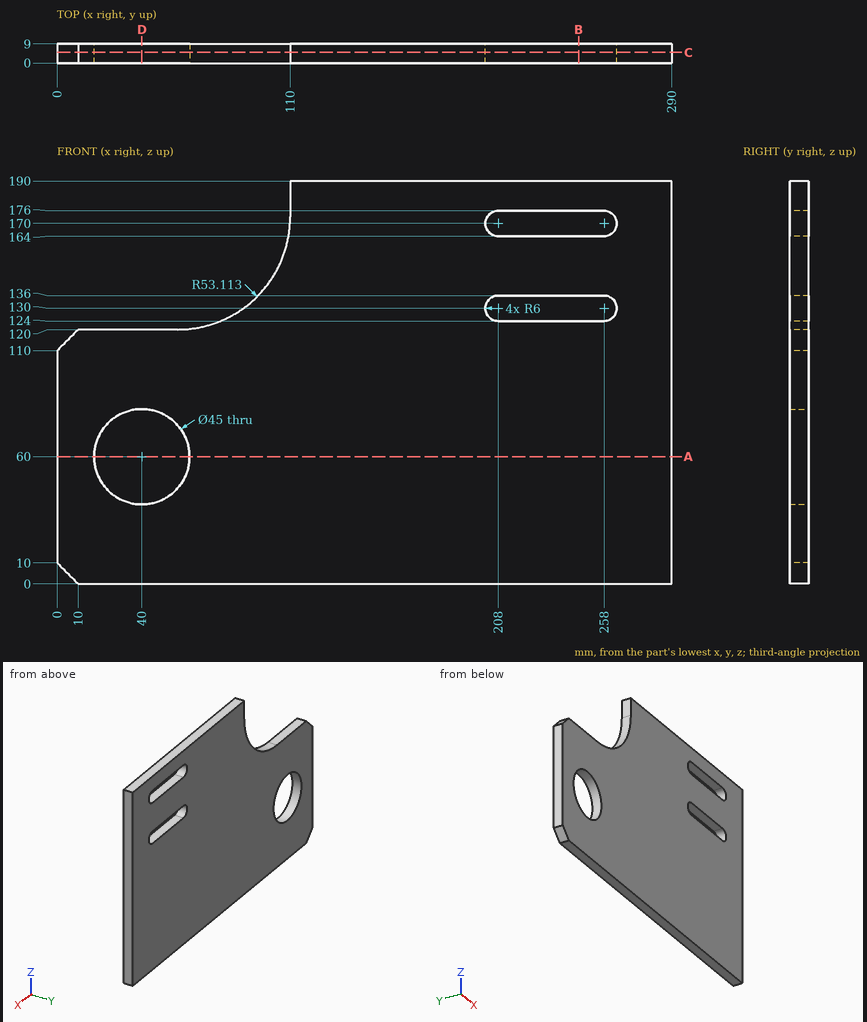
Study the drawing (mm; zero at the part's minimum x, y, z) and answer. Give positions to 0.01 mm unless a question says otherwise; leave off trailing zeros. Write each loop counter-clockwise with the first axis right and the second up, starting at its lowest first coordinate (ties: lowest second). Pieces come first, ordered by that corner, then holes. Notation, with made-up numbers: (51, 74) -> (76, 74) arc R10 cw to (76, 88) -> close; hole circle Ø8 at (26, 1.25). An arc over 180 degrees is marked (long way). Answer as a JSON object with one key per item and string values. Group by question number.
1) Find section C-C (y = 5). Write down the section's boundary in (x, z) (1 decimal), and give its area (3 significant figures).
2) Find section B-B (x = 246). Write down the section's boundary in (y, z).
3) This flat-tipped pin is pushed along its axis until it touches: P1, Ø4.5, axis at y = 2.5, z = 180.5, coming from the -X side. Where does it stop, or does it pass through?
4) Find section D-D (x = 40). Write down the section's boundary in (y, z), and give its area (3 significant figures).
5) Consider L1, parallel to Z at x = 247, y = 1; L2, parallel to Z at x = 40, y = 5.25; L3, parallel to Z at x = 207, y = 6.75. Determine where each line is inside the solid, lowest interval first. Write a range as from..to.
6) Find section A-A (z = 60). Write down the section's boundary in (x, y), and give its area (4 significant figures).
Values follow:
{
 "1": {"outline": "(0, 10) -> (10, 0) -> (290, 0) -> (290, 190) -> (110, 190) -> (110, 173.1) arc R53.1 cw to (56.9, 120) -> (10, 120) -> (0, 110) -> close; hole circle Ø45 at (40, 60); hole (208, 124) -> (258, 124) arc R6 ccw to (258, 136) -> (208, 136) arc R6 ccw to start; hole (208, 164) -> (258, 164) arc R6 ccw to (258, 176) -> (208, 176) arc R6 ccw to start", "area": "44,900 mm2"},
 "2": {"outline": "(0, 0) -> (9, 0) -> (9, 124) -> (0, 124) -> close; (0, 136) -> (9, 136) -> (9, 164) -> (0, 164) -> close; (0, 176) -> (9, 176) -> (9, 190) -> (0, 190) -> close"},
 "3": {"P1": "stops at x = 110"},
 "4": {"outline": "(0, 0) -> (9, 0) -> (9, 37.5) -> (0, 37.5) -> close; (0, 82.5) -> (9, 82.5) -> (9, 120) -> (0, 120) -> close", "area": "675 mm2"},
 "5": {"L1": "z = 0..124, 136..164, 176..190", "L2": "z = 0..37.5, 82.5..120", "L3": "z = 0..124.08, 135.92..164.08, 175.92..190"},
 "6": {"outline": "(0, 0) -> (17.5, 0) -> (17.5, 9) -> (0, 9) -> close; (62.5, 0) -> (290, 0) -> (290, 9) -> (62.5, 9) -> close", "area": "2,205 mm2"}
}
